```python
from build123d import *

# Parameters (mm, degrees)
F0_R     = 21
F1_DEPTH = 100
F2_SIZE  = 1
F3_R     = 4
F4_DEPTH = 100.001


with BuildPart() as f1:
    # F0 (on Front) → F1 (new body)
    with BuildSketch(Plane.XZ):
        Circle(F0_R)
    extrude(amount=F1_DEPTH)

    # F2
    f2_edges = [f1.edges().sort_by_distance(p)[0] for p in [
        (-21, 0, 0),
    ]]
    chamfer(f2_edges, length=F2_SIZE)

    # F3 (on face) → F4 (cut, through all)
    with BuildSketch(Plane(origin=(0, 0, 0), x_dir=(-1, 0, 0), z_dir=(0, 1, 0))):
        Circle(F3_R)
    extrude(amount=-F4_DEPTH, mode=Mode.SUBTRACT)


solid = f1.part
```
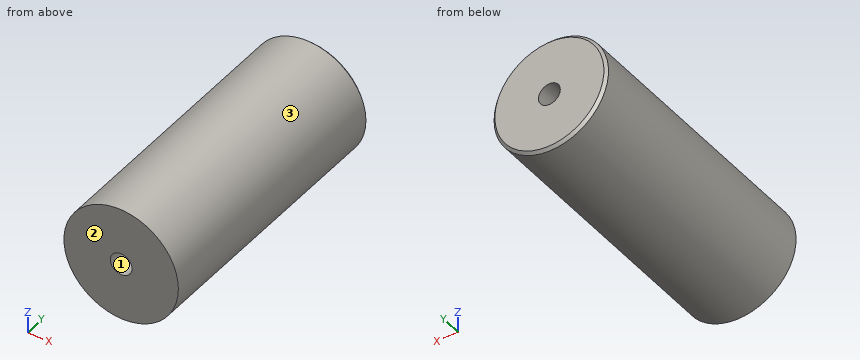
Could you check a few things on this model? Use its own coordinates, in mm. Face numbers are marked on the shaded views. Round coordinates to 2 decimals unless told otherwise and drop trailing zeros. Write each loop counter-clockwise with the first axis right and the second up, starting at its lowest first coordinate (ties: lowest second). Pieces come first, ordered by that corner, then holes.
(1) Thinking about a two-plate mould opening in X: for the marked faces 1, 2 and 3, which applies, +X half, -X half, draft (parallel to the pull), parting line (faces both ways), or undercut?
Findings below:
face 1: undercut
face 2: draft
face 3: parting line
(2) Suppose I cut it at C-C on y = -16.5. Write out the boundary of the cut face in (x, z).
Findings below:
outline: circle Ø42 at (0, 0); hole circle Ø8 at (0, 0)
(3) For pin 1 (2 mm diameter, centred on y = -45.5, z = -10, fed in from -X); pin 2 (8 mm diameter, centred on x = -6.5, y = -27, fed in from +Z); pin 3 (8 mm diameter, centred on x = -2, y = -25, fed in from +Z), each with a flat end and sliding along its axis, tell me the tip position at first contact or that it passes through.
Findings below:
pin 1: stops at x = -18.97
pin 2: stops at z = 20.85
pin 3: stops at z = 21
(4) Suppose I cut it at B-B on z = 0. Write out the boundary of the cut face in (x, y).
Findings below:
outline: (-21, -100) - (-4, -100) - (-4, 0) - (-20, 0) - (-21, -1) - close; (4, -100) - (21, -100) - (21, -1) - (20, 0) - (4, 0) - close
(5) Suppose I cut it at A-A on x = 0. Write out the boundary of the cut face in (y, z), and give its area (3 significant figures).
Findings below:
outline: (-100, -21) - (-1, -21) - (0, -20) - (0, -4) - (-100, -4) - close; (-100, 4) - (0, 4) - (0, 20) - (-1, 21) - (-100, 21) - close
area: 3,400 mm2
(6) If I drill on probe 1 along Z at (x, y) = (0, -51); probe 2 along Z at (x, y) = (-3, -57); probe 3 along X at (y, z) = (-75.5, 2), over which ranges is the centre line in solid material (lowest first)?
Findings below:
probe 1: z = -21 to -4, 4 to 21
probe 2: z = -20.78 to -2.65, 2.65 to 20.78
probe 3: x = -20.9 to -3.46, 3.46 to 20.9
